```python
from build123d import *

# Parameters (mm, degrees)
SKETCH2_W                               = 300
SKETCH2_H                               = 200
BOSS_EXTRUDE1_DEPTH                     = 20
SKETCH3_W                               = 280
SKETCH3_H                               = 180
SKETCH3_W_2                             = 270
SKETCH3_H_2                             = 170
BOSS_EXTRUDE2_DEPTH                     = 10
FILLET1_R                               = 40
FILLET2_R                               = 60
SKETCH4_R                               = 39
CUT_EXTRUDE1_DEPTH                      = 16
SKETCH5_R                               = 32.5
CUT_EXTRUDE2_DEPTH                      = 16
SKETCH8_R                               = 1.5
CUT_EXTRUDE3_DEPTH                      = 20
CBORE_FOR_M5_HEX_HEAD_BOLT1_D           = 3
CBORE_FOR_M5_HEX_HEAD_BOLT1_DEPTH       = 20
CBORE_FOR_M5_HEX_HEAD_BOLT1_CBORE_D     = 5.2
CBORE_FOR_M5_HEX_HEAD_BOLT1_CBORE_DEPTH = 1.7
CBORE_FOR_M5_HEX_HEAD_BOLT1_TIP         = 0.901290929


with BuildPart() as part:
    # Sketch2 → Boss-Extrude1 (new body)
    with BuildSketch(Plane(origin=(0, 0, 0), x_dir=(1, 0, 0), z_dir=(0, 1, 0))):
        Rectangle(SKETCH2_W, SKETCH2_H)
    extrude(amount=BOSS_EXTRUDE1_DEPTH)

    # Sketch3 → Boss-Extrude2 (add)
    with BuildSketch(Plane.XZ):
        Rectangle(SKETCH3_W, SKETCH3_H)
        Rectangle(SKETCH3_W_2, SKETCH3_H_2, mode=Mode.SUBTRACT)
    extrude(amount=BOSS_EXTRUDE2_DEPTH)

    # Fillet1
    fillet1_edges = [part.edges().sort_by_distance(p)[0] for p in [
        (140, -5, -90),
        (140, -5, 90),
        (135, -5, -85),
        (135, -5, 85),
        (150, 10, -100),
        (150, 10, 100),
    ]]
    fillet(fillet1_edges, radius=FILLET1_R)

    # Fillet2
    fillet2_edges = [part.edges().sort_by_distance(p)[0] for p in [
        (-140, -5, 90),
        (-140, -5, -90),
        (-135, -5, -85),
        (-135, -5, 85),
        (-150, 10, -100),
        (-150, 10, 100),
    ]]
    fillet(fillet2_edges, radius=FILLET2_R)

    # Sketch4 → Cut-Extrude1 (cut)
    with BuildSketch(Plane(origin=(0, 20, 0), x_dir=(1, 0, 0), z_dir=(0, 1, 0))):
        with Locations(Location((90, 0, 0), (0, 0, 270))):
            Circle(SKETCH4_R)
    extrude(amount=-CUT_EXTRUDE1_DEPTH, mode=Mode.SUBTRACT)

    # Sketch5 → Cut-Extrude2 (cut)
    with BuildSketch(Plane(origin=(0, 4, 0), x_dir=(1, 0, 0), z_dir=(0, 1, 0))):
        with Locations(Location((90, 0, 0), (0, 0, 270))):
            Circle(SKETCH5_R)
    extrude(amount=-CUT_EXTRUDE2_DEPTH, mode=Mode.SUBTRACT)

    # Sketch8 → Cut-Extrude3 (cut)
    with BuildSketch(Plane.XZ):
        with Locations(Location((-100, 92, 0), (0, 0, 270))):
            Circle(SKETCH8_R)
        with Locations(Location((-100, -92, 0), (0, 0, 270))):
            Circle(SKETCH8_R)
        with Locations(Location((-145, 35, 0), (0, 0, 270))):
            Circle(SKETCH8_R)
        with Locations(Location((-145, -35, 0), (0, 0, 270))):
            Circle(SKETCH8_R)
        with Locations(Location((110, 94, 0), (0, 0, 270))):
            Circle(SKETCH8_R)
        with Locations(Location((110, -94, 0), (0, 0, 270))):
            Circle(SKETCH8_R)
        with Locations(Location((145, 35, 0), (0, 0, 270))):
            Circle(SKETCH8_R)
        with Locations(Location((145, -35, 0), (0, 0, 270))):
            Circle(SKETCH8_R)
    extrude(amount=-CUT_EXTRUDE3_DEPTH, mode=Mode.SUBTRACT)

    # CBORE for M5 Hex Head Bolt1
    with Locations(Plane(origin=(0, 20, 0), x_dir=(1, 0, 0), z_dir=(0, 1, 0))):
        with Locations((110, 94), (145, 35), (145, -35), (110, -94), (-100, -92), (-145, -35), (-145, 35), (-100, 92)):
            CounterBoreHole(CBORE_FOR_M5_HEX_HEAD_BOLT1_D / 2, CBORE_FOR_M5_HEX_HEAD_BOLT1_CBORE_D / 2, CBORE_FOR_M5_HEX_HEAD_BOLT1_CBORE_DEPTH, depth=CBORE_FOR_M5_HEX_HEAD_BOLT1_DEPTH)
            with Locations((0, 0, -(CBORE_FOR_M5_HEX_HEAD_BOLT1_DEPTH + CBORE_FOR_M5_HEX_HEAD_BOLT1_TIP / 2))):  # 118° drill point
                Cone(0, CBORE_FOR_M5_HEX_HEAD_BOLT1_D / 2, CBORE_FOR_M5_HEX_HEAD_BOLT1_TIP, mode=Mode.SUBTRACT)


solid = part.part
```
Source: CAD feature listing. Evaluate the final solid. Frame: model axes, mm. A direction names the side the tool comes from. Round coordinates to 2 decimals unless told otherwise and drop trailing zeros. Write each loop counter-clockwise with the first axis right and the second up, starting at its lowest first coordinate (ties: lowest second). Pieces come first, ordered by that corner, then holes. Notation, with made-up numbers: M 68.5,32 L 83.5,32 A22 ccw 83.5,56 Z; hole C -32,21.25 d2. An arc over 180 degrees is marked long. Use CSV: the item, a comma, the result in double quotes. Start each with the question number.
Q1. Access query for faces 4 (the face through (-121.96, -5.07, 72.89)), 5 (the face through (-116.96, -5.07, -67.89)), 6 (the face through (9, -5, -90)). Directions: +Z, -Z, +X, -X, +Y, -Y. A direction counts if a zero-diameter tool reaches every point of the face in a straight line with its end or side. Return the directions, or none.
Q2. Cut plane B-B on z = 1.5. Output: boundary loops of the cut face in (x, y), plus the area to 3 significant figures.
Q3. Pull-direction query (X, two-part tool) for faces 1 (the face through (9, -5, 85)), 2 (the face through (-140, -5, 0)), 3 (the face through (127.972, -5.07, 78.594)); classes: +X half, -X half, draft (parallel to the pull), parting line (faces both ways), or undercut.
Q4. Line query: line 1 (X direction, y = 0.9, z = 0); line 2 (X direction, y = 18.8, z = 35); line 3 (Z direction, x = -9, y = -8.25). Output: solid intervals per line, ascending. Write a range as from..to.
Q5. Cut plane C-C on x = 117. Output: boundary loops of the cut face in (y, z).
Q6. First-contact query: P1, Ø3.5, axis at x = 110, z = 94, coming from the -Y side; P2, Ø5, axis at y = -4, z = -24, coming from the +X side; P3, Ø8, axis at y = 16.5, z = 73, coming from the +X side. Flat tips, straight axial feed; report the tip coordinate or a pass-through.
Q7. Cut plane D-D on y = 13. Count the separate pieces of the cut face and the enclosed holes in it, plus the area to 3 significant figures.
Q8. Cut plane A-A on y = -5.5. Output: boundary loops of the cut face in (x, z), plus the area to 3 significant figures.
Results found:
1,face 4,"+Z, -X, -Y"
1,face 5,"-Y"
1,face 6,"-Z, +X, -X, -Y"
2,outline,"M -150,0 L -140,0 L -140,-10 L -135,-10 L -135,0 L 57.53,0 L 57.53,4 L 51.03,4 L 51.03,20 L -150,20 Z; M 122.47,0 L 135,0 L 135,-10 L 140,-10 L 140,0 L 150,0 L 150,20 L 128.97,20 L 128.97,4 L 122.47,4 Z"
2,area,"4,590 mm^2"
3,face 1,"undercut"
3,face 2,"-X half"
3,face 3,"+X half"
4,line 1,"-150..57.5, 122.5..150"
4,line 2,"-150..-147.6, -142.4..72.8, 107.2..142.4, 147.6..150"
4,line 3,"-90..-85, 85..90"
5,outline,"M -10,-86.21 L 0,-86.21 L 0,-99.38 L 20,-99.38 L 20,-28.14 L 4,-28.14 L 4,-18.09 L 0,-18.09 L 0,-78.41 L -10,-78.41 Z; M -10,78.41 L 0,78.41 L 0,18.09 L 4,18.09 L 4,28.14 L 20,28.14 L 20,99.38 L 0,99.38 L 0,86.21 L -10,86.21 Z"
6,P1,"y = 0"
6,P2,"x = 140"
6,P3,"x = 148.97"
7,separate pieces,"1"
7,enclosed holes,"9"
7,area,"52,900 mm^2"
8,outline,"M -140,-30 A60 ccw -80,-90 L 100,-90 A40 ccw 140,-50 L 140,50 A40 ccw 100,90 L -80,90 A60 ccw -140,30 Z; hole M -135,-25 A60 ccw -75,-85 L 95,-85 A40 ccw 135,-45 L 135,45 A40 ccw 95,85 L -75,85 A60 ccw -135,25 Z"
8,area,"4,500 mm^2"
